CAD build for the part. Positions are in the model's coordinates, mm. A direction names the side the tool comes from. Coordinates: 2 decimals unless noted, no trailing zeros. Loops run counter-clockwise (first coordinate to the right, second up) from the corner with the lowest first, then second, coordinate; pieces in that order, holes last. Notation, with made-up numbers: (21.25, -38) -> (75.25, -38) arc R24 cw to (75.25, -17) -> close; hole circle Ø1 at (78.25, -29). An arc over 180 degrees is marked (long way). Write item = value, one per line. Start each with the question number.
(1) Band-saw the part on A-A (x = 0). Count the separate pieces of the cut face and the enclosed holes in it, and give its area (3 significant figures).
(2) Drill centre lines: line 1 (Z direction, x = 0, y = 46.55); line 2 (Y direction, x = 12, z = 12.5); line 3 (Z direction, x = 0, y = 22). Where is each one in solid material? Low to high. Write a range as from..to.
(3) Band-saw the part on B-B (z = 0). Write the cut outline in (x, y), and give its area (3 significant figures).
(4) Band-saw the part on C-C (z = -17.25). Write the cut outline in (x, y).
(5) Tool access for faces 1 (the face through (10, 44.5, 10)), 2 (the face through (-0.5, 2.2, -19.7)): list every direction of +Z, -Z, +X, -X, +Y, -Y with a clear straight run to the whole face (end or side of a thin tool).
(6) Pull direction X, two halves, no side cores. Call faces 3 (the face through (10.382, 2.218, 19.961)), 4 (the face through (-0.867, 24.157, -3.905)), 5 (the face through (5, 0, 0)): +X half, -X half, draft (parallel to the pull), parting line (faces both ways), or undercut.
(7) Flat gauge pins, fed straight in: P1, Ø8, axis at x = -3.5, y = 31.5, coming from the -Z side; P2, Ø10, axis at x = 7.5, y = 19, coming from the -Z side; P3, Ø3, axis at x = -10.5, y = 43.5, coming from the -Z side. Where does each tip first touch, or does it go through?
(8) Band-saw the part on D-D (z = 7.5). Write the cut outline in (x, y).
```python
from build123d import *

# Parameters (mm, degrees)
SKETCH1_R           = 22.5
BOSS_EXTRUDE1_DEPTH = 4.5
SKETCH2_R           = 12
BOSS_EXTRUDE2_DEPTH = 40
SKETCH3_R           = 22.5
BOSS_EXTRUDE3_DEPTH = 4.5
SKETCH4_R           = 4
CUT_EXTRUDE1_DEPTH  = 60.5
SKETCH5_R           = 2.5
CUT_EXTRUDE2_DEPTH  = 60.5


with BuildPart() as part:
    # Sketch1 → Boss-Extrude1 (new body)
    with BuildSketch(Plane(origin=(0, 0, 0), x_dir=(1, 0, 0), z_dir=(0, 1, 0))):
        Circle(SKETCH1_R)
    extrude(amount=BOSS_EXTRUDE1_DEPTH)

    # Sketch2 → Boss-Extrude2 (add)
    with BuildSketch(Plane(origin=(0, 4.5, 0), x_dir=(1, 0, 0), z_dir=(0, 1, 0))):
        Circle(SKETCH2_R)
    extrude(amount=BOSS_EXTRUDE2_DEPTH)

    # Sketch3 → Boss-Extrude3 (add)
    with BuildSketch(Plane(origin=(0, 44.5, 0), x_dir=(1, 0, 0), z_dir=(0, 1, 0))):
        Circle(SKETCH3_R)
    extrude(amount=BOSS_EXTRUDE3_DEPTH)

    # Sketch4 → Cut-Extrude1 (cut)
    with BuildSketch(Plane.XZ):
        Circle(SKETCH4_R)
    extrude(amount=-CUT_EXTRUDE1_DEPTH, mode=Mode.SUBTRACT)

    # Sketch5 → Cut-Extrude2 (cut)
    with BuildSketch(Plane.XZ):
        with Locations((0, 17.25)):
            Circle(SKETCH5_R)
        with Locations((14.938938215, 8.625)):
            Circle(SKETCH5_R)
        with Locations((14.938938215, -8.625)):
            Circle(SKETCH5_R)
        with Locations((0, -17.25)):
            Circle(SKETCH5_R)
        with Locations((-14.938938215, -8.625)):
            Circle(SKETCH5_R)
        with Locations((-14.938938215, 8.625)):
            Circle(SKETCH5_R)
    extrude(amount=-CUT_EXTRUDE2_DEPTH, mode=Mode.SUBTRACT)


solid = part.part
```
Findings below:
q1.separate_pieces = 6
q1.enclosed_holes = 0
q1.area = 883 mm²
q2.line_1 = -22.5..-19.75, -14.75..-4, 4..14.75, 19.75..22.5
q2.line_2 = 0..4.5, 44.5..49
q2.line_3 = -12..-4, 4..12
q3.outline = (-22.5, 0) -> (-4, 0) -> (-4, 49) -> (-22.5, 49) -> (-22.5, 44.5) -> (-12, 44.5) -> (-12, 4.5) -> (-22.5, 4.5) -> close; (4, 0) -> (22.5, 0) -> (22.5, 4.5) -> (12, 4.5) -> (12, 44.5) -> (22.5, 44.5) -> (22.5, 49) -> (4, 49) -> close
q3.area = 973 mm²
q4.outline = (-14.45, 0) -> (-2.5, 0) -> (-2.5, 4.5) -> (-14.45, 4.5) -> close; (-14.45, 44.5) -> (-2.5, 44.5) -> (-2.5, 49) -> (-14.45, 49) -> close; (2.5, 0) -> (14.45, 0) -> (14.45, 4.5) -> (2.5, 4.5) -> close; (2.5, 44.5) -> (14.45, 44.5) -> (14.45, 49) -> (2.5, 49) -> close
q5.face_1 = none
q5.face_2 = +Y, -Y
q6.face_3 = parting line
q6.face_4 = undercut
q6.face_5 = draft
q7.P1 = -12
q7.P2 = -11.74
q7.P3 = -20.45
q8.outline = (-21.21, 0) -> (-17.17, 0) -> (-17.17, 4.5) -> (-21.21, 4.5) -> close; (-21.21, 44.5) -> (-17.17, 44.5) -> (-17.17, 49) -> (-21.21, 49) -> close; (-12.71, 0) -> (12.71, 0) -> (12.71, 4.5) -> (9.37, 4.5) -> (9.37, 44.5) -> (12.71, 44.5) -> (12.71, 49) -> (-12.71, 49) -> (-12.71, 44.5) -> (-9.37, 44.5) -> (-9.37, 4.5) -> (-12.71, 4.5) -> close; (17.17, 0) -> (21.21, 0) -> (21.21, 4.5) -> (17.17, 4.5) -> close; (17.17, 44.5) -> (21.21, 44.5) -> (21.21, 49) -> (17.17, 49) -> close
